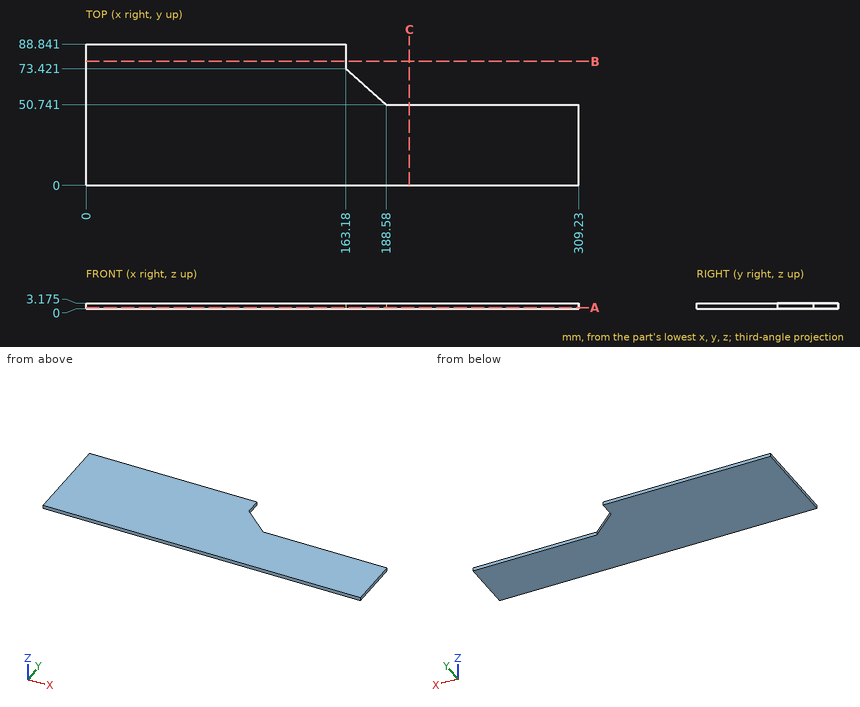
Geometry check sheet. Reference: drawing and pictorial views, mm from the part's lowest x, y, z. Coordinates: 2 decimals unless noted, no trailing zeros. Loops run counter-clockwise (first coordinate to the right, second up) from the corner with the lowest first, then second, coordinate; pieces in that order, holes last. Notation, with made-up numbers: M -29,-20.75 L -24,-20.75 A19 ccw -24,8.25 Z; hole C 58,3 d10. An arc over 180 degrees is marked long. One line per item, written item: value.
1. Gauge pin test, flat end, axial feed: P1, Ø1, axis at y = 83.5, z = 1, coming from the +X side. Record the tip position at first contact, or that the pin passes through.
Answers follow:
P1: x = 163.18
2. Section check C-C on x = 203. Record the cut outline in (y, z) (3 decimals).
Answers follow:
outline: M 0,0 L 50.741,0 L 50.741,3.175 L 0,3.175 Z
3. Material ranges on line 1 along Y through (x, z) = (215, 1.75); line 2 along X through (y, z) = (77.5, 2.7); line 3 along Y through (x, z) = (174.5, 1.8), recorded low to high. Write a range as from..to.
Answers follow:
line 1: 0..50.74
line 2: 0..163.18
line 3: 0..63.31
4. Section check B-B on y = 78. Record the cut outline in (x, z) (3 decimals), plus the area to 3 significant figures.
Answers follow:
outline: M 0,0 L 163.18,0 L 163.18,3.175 L 0,3.175 Z
area: 518 mm^2
5. Section check A-A on z = 0.6. Record the cut outline in (x, y).
Answers follow:
outline: M 0,0 L 309.23,0 L 309.23,50.74 L 188.58,50.74 L 163.18,73.42 L 163.18,88.84 L 0,88.84 Z
